Can you work these out from the model? Positions are in its coordinate system, mm. Face numbers are marked on the shaded views. A direction names the side the tool comes from. Give positions to 0.01 mm unless a question says otherwise; leave off trailing zeros. Order: outer loops, then holes, each group sorted by start corner. A loop starts at its lowest first (then second) coordinate and runs counter-clockwise, first axis right, second up. Notation, with made-up numbers: (9.5, 11.25) -> (13.5, 11.25) arc R15 ccw to (13.5, 26.25) -> close; hole circle Ø7 at (30.5, 1). An arc over 180 degrees is marked (long way). Answer as CSV lines item,"result".
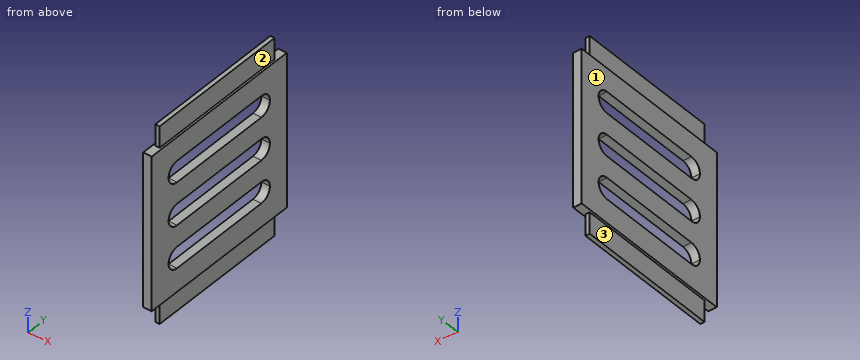
Autodesk Inventor part; units mm, degrees
ref_plane "YZ Plane" through (0, 0, 0) normal (1, 0, 0) x (0, 1, 0)
ref_plane "XZ Plane" through (0, 0, 0) normal (0, 1, 0) x (-1, 0, 0)
ref_plane "XY Plane" through (0, 0, 0) normal (0, 0, 1) x (1, 0, 0)
sketch "Sketch1" plane through (0, 0, 0) normal (0, 1, 0) x (-1, 0, 0)
  line L0 (0, 0) -> (10, 0)
  line L1 (10, 0) -> (10, -180)
  line L2 (10, -180) -> (0, -180)
  line L3 (0, -180) -> (0, 0)
  dimension "d0" = 10
  dimension "d1" = 180
extrude "Extrusion1" add sketch "Sketch1" along normal blind 200
sketch "Sketch2" plane through (-10, 0, 0) normal (0, 0, 1) x (1, 0, 0)
  line L0 (10, 0) -> (0, 0)
  line L1 (10, 200) -> (0, 200)
  line L2 (2.5, 0) -> (7.5, 0)
  line L3 (7.5, 0) -> (7.5, 200)
  line L4 (7.5, 200) -> (2.5, 200)
  line L5 (2.5, 200) -> (2.5, 0)
  line L6 (10, 0) -> (10, 200)
  line L7 (0, 200) -> (10, 200)
  line L8 (10, 200) -> (10, 185)
  line L9 (10, 185) -> (0, 185)
  line L10 (0, 185) -> (0, 200)
  line L11 (0, 0) -> (10, 0)
  line L12 (10, 0) -> (10, 15)
  line L13 (10, 15) -> (0, 15)
  line L14 (0, 15) -> (0, 0)
  point P0 (2.5, 15)
  point P1 (7.5, 15)
  point P2 (7.5, 185)
  point P3 (2.5, 185)
  dimension "d4" = 5
  dimension "d5" = 15
  dimension "d6" = 15
extrude "Extrusion2" add sketch "Sketch2" along normal blind 25 contours L13 L5 L9 L3
sketch "Sketch3" plane through (0, 0, -180) normal (0, 0, -1) x (-1, 0, 0)
  line L0 (2.5, 15) -> (7.5, 15)
  line L1 (7.5, 15) -> (7.5, 185)
  line L2 (7.5, 185) -> (2.5, 185)
  line L3 (2.5, 185) -> (2.5, 15)
  point P0 (0, 0)
  dimension "d9" = 5
  dimension "d10" = 170
extrude "Extrusion3" add sketch "Sketch3" along normal blind 25
sketch "Sketch4" plane through (0, 0, 0) normal (1, 0, 0) x (0, 0, -1)
  line L0 (27.5, 175) -> (52.5, 175)
  line L1 (52.5, 175) -> (52.5, 25)
  line L2 (52.5, 25) -> (27.5, 25)
  line L3 (27.5, 25) -> (27.5, 175)
  line L4 (77.5, 25) -> (102.5, 25)
  line L5 (102.5, 25) -> (102.5, 175)
  line L6 (102.5, 175) -> (77.5, 175)
  line L7 (77.5, 175) -> (77.5, 25)
  line L8 (127.5, 175) -> (152.5, 175)
  line L9 (152.5, 175) -> (152.5, 25)
  line L10 (152.5, 25) -> (127.5, 25)
  line L11 (127.5, 25) -> (127.5, 175)
  point P0 (0, 0)
  dimension "d13" = 25
  dimension "d14" = 150
  dimension "d15" = 25
  dimension "d16" = 25
extrude "Extrusion4" cut sketch "Sketch4" against normal blind 10
fillet "Fillet1" radius 12.5 12 edges at (-5, 175, -77.5) (-5, 175, -102.5) (-5, 175, -152.5) (-5, 175, -127.5) (-5, 175, -27.5) (-5, 175, -52.5) (-5, 25, -102.5) (-5, 25, -52.5) (-5, 25, -27.5) (-5, 25, -77.5) (-5, 25, -127.5) (-5, 25, -152.5)
properties part number "TSU_MM_Wall"
Item 1: Imagine slicing it at A-A, the plane y = 145. Please give me the cut outline in (x, z).
Numbers:
outline,"(-10, -180) -> (-7.5, -180) -> (-7.5, -205) -> (-2.5, -205) -> (-2.5, -180) -> (0, -180) -> (0, -152.5) -> (-10, -152.5) -> close; (-10, -127.5) -> (0, -127.5) -> (0, -102.5) -> (-10, -102.5) -> close; (-10, -77.5) -> (0, -77.5) -> (0, -52.5) -> (-10, -52.5) -> close; (-10, -27.5) -> (0, -27.5) -> (0, 0) -> (-2.5, 0) -> (-2.5, 25) -> (-7.5, 25) -> (-7.5, 0) -> (-10, 0) -> close"
Item 2: Imagine slicing it at C-C, the plane x = -4.75. Give the number of separate pieces and of enclosed holes in the cut face, then the cut area to 3 significant figures.
Numbers:
separate pieces,"1"
enclosed holes,"3"
area,"33,700 mm²"
Item 3: Please list where these lines run through material, in increasing order: line 1 along Z through (x, y) = (-8.75, 115.5); line 2 along Z through (x, y) = (-7.25, 118); line 3 along Y through (x, z) = (-2, -41.5).
Numbers:
line 1,"z = -180 to -152.5, -127.5 to -102.5, -77.5 to -52.5, -27.5 to 0"
line 2,"z = -205 to -152.5, -127.5 to -102.5, -77.5 to -52.5, -27.5 to 25"
line 3,"y = 0 to 25.09, 174.91 to 200"
Item 4: For the marked faces 1, 2 and 3, which set-ups out of +Z, -Z, +X, -X, +Y, -Y let a thin tool reach every point of the face, with its end or its side?
Numbers:
face 1,"+Z, -Z, -X, +Y, -Y"
face 2,"+Z, +X, +Y, -Y"
face 3,"-Z, -X, +Y, -Y"
Item 5: Imagine slicing it at D-D, the plane z = -188. Please give me the cut outline in (x, y), then the cut area to 3 significant figures.
Numbers:
outline,"(-7.5, 15) -> (-2.5, 15) -> (-2.5, 185) -> (-7.5, 185) -> close"
area,"850 mm²"
Item 6: For pin 1 (1.5 mm diameter, centred on x = -5.5, z = -187.5, fed in from +Y); pin 2 (7.5 mm diameter, centred on y = 88.5, z = 8.5, fed in from -X); pin 3 (10 mm diameter, centred on y = 62.5, z = -84, fed in from +X), each with a flat end and sliding along its axis, tell me the tip position at first contact or that it passes through.
Numbers:
pin 1,"stops at y = 185"
pin 2,"stops at x = -7.5"
pin 3,"passes through"
Item 7: Imagine slicing it at B-B, the plane z = -133. Please give me the cut outline in (x, y), then the cut area to 3 significant figures.
Numbers:
outline,"(-10, 0) -> (0, 0) -> (0, 27.14) -> (-10, 27.14) -> close; (-10, 172.86) -> (0, 172.86) -> (0, 200) -> (-10, 200) -> close"
area,"543 mm²"
